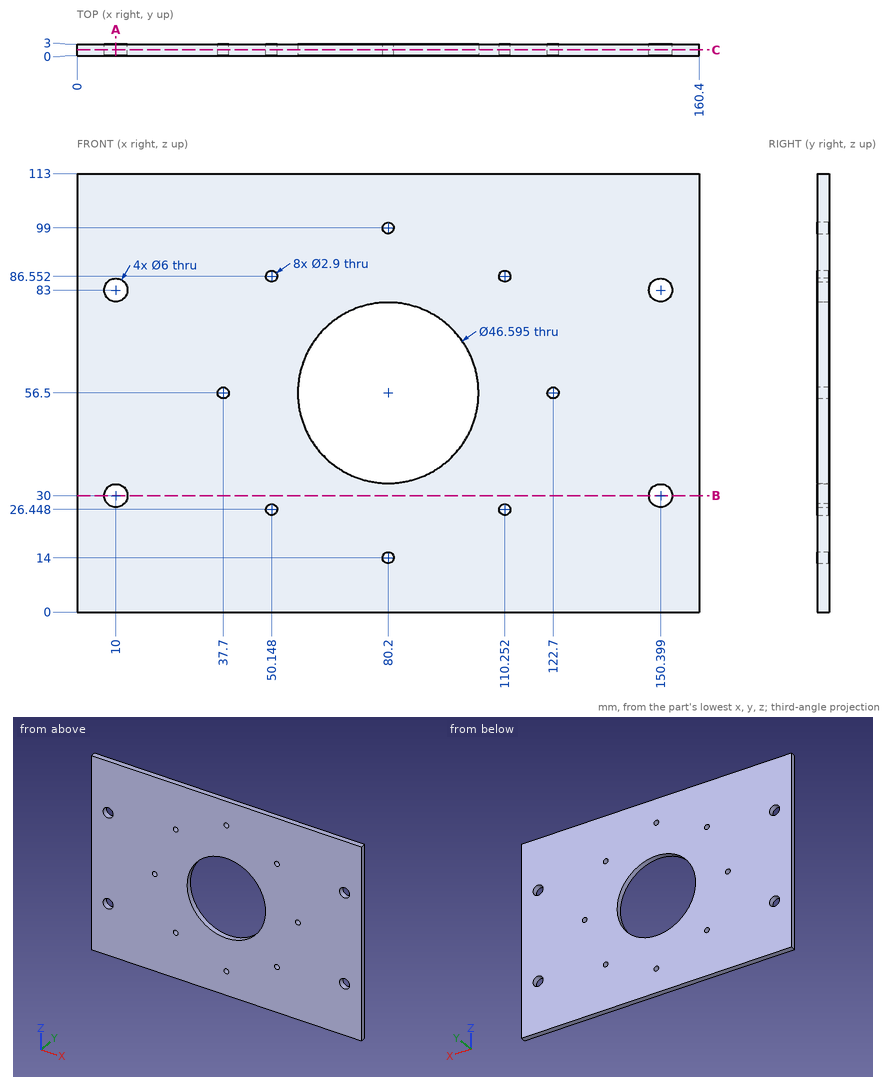
The figure shows three views and two pictorial views of one solid part (mm, origin at its lowest corner). Answer the questions. Give positions to 0.01 mm unless a question says otherwise; leave off trailing zeros. Order: outer loops, then holes, each group sorted by start corner. A loop starts at its lowest first (then second) coordinate and runs counter-clockwise, first axis right, second up. Notation, with made-up numbers: (-31, 20) -> (2, 20) arc R21 cw to (2, 53) -> close; hole circle Ø5 at (-13.5, 24). An arc over 180 degrees is marked (long way). Answer as CSV lines item,"result". Start each with the question number.
Q1. A cutting plane is placed at C-C (y = 1.5). Count the separate pieces of the cut face and the enclosed holes in it, then the cut area to 3 significant figures.
Q2. Find the intervals of material crossed by L1, parallel to X at y = 1.6, z = 56.5; L2, parallel to Z at x = 150.5, y = 0.7; L3, parallel to X at y = 0.7, z = 30, in increasing order.
Q3. A cutting plane is placed at B-B (z = 30). Determine the outline of the cut face in (x, y).
Q4. Given pin 1 (4 mm diameter, centred on x = 75, z = 91.5, fed in from -Y), flat-ended and moving along its own axis, determine where the tip first touches the part or whether it passes through.
Q5. A cutting plane is placed at A-A (x = 10). Determine the outline of the cut face in (y, z), then the cut area to 3 significant figures.
Results found:
1,separate pieces,"1"
1,enclosed holes,"13"
1,area,"16,300 mm2"
2,L1,"0 to 36.25, 39.15 to 56.9, 103.5 to 121.25, 124.15 to 160.4"
2,L2,"0 to 27, 33 to 80, 86 to 113"
2,L3,"0 to 7, 13 to 147.4, 153.4 to 160.4"
3,outline,"(0, 0) -> (7, 0) -> (7, 3) -> (0, 3) -> close; (13, 0) -> (147.4, 0) -> (147.4, 3) -> (13, 3) -> close; (153.4, 0) -> (160.4, 0) -> (160.4, 3) -> (153.4, 3) -> close"
4,pin 1,"y = 0"
5,outline,"(0, 0) -> (3, 0) -> (3, 27) -> (0, 27) -> close; (0, 33) -> (3, 33) -> (3, 80) -> (0, 80) -> close; (0, 86) -> (3, 86) -> (3, 113) -> (0, 113) -> close"
5,area,"303 mm2"
